Could you check a few things on this drawing? It's one solid part, dimensions in mm from its lowest x, y, z. A direction names the side the tool comes from. Round coordinates to 2 decimals unless told otherwise and drop trailing zeros. Order: outer loops, then holes, each group sorted by start corner. A loop starts at its lowest first (then second) coordinate and runs counter-clockwise, first axis right, second up. Notation, with made-up numbers: (64, 31.25) -> (79, 31.25) arc R30 cw to (79, 67.25) -> close; hole circle Ø6 at (35, 22). An arc over 180 degrees is marked (long way). Use a Markdown table: item, result. Add a question column.
(1) If I drill on probe 1 along X at (y, z) = (5.75, 6.5); probe 2 along X at (y, z) = (0.8, 5) (1 decimal); probe 3 along X at (y, z) = (0.55, 30) (1 decimal), over which ranges is the centre line in solid material (lowest first)?
(2) I want a section at B-B, the plane y = 8.25. Please give me the cut outline in (x, z).
(3) Thinking about a two-plate mould opening in X: for the marked faces 5, 6, 7 and 8, which applies, pulls with the +X half, pulls with the -X half, needs draft (parallel to the pull), parting line crosses it, or undercut?
(4) On a 3-axis mill with a long thin cutter (end or side, diameter ignored), from which of +Z, -Z, +X, -X, +Y, -Y can I reach the whole of each face in a straight line? I mean the marked faces 1, 2, 3 and 4. Say none if no direction works.
(5) I want a section at D-D, the plane z = 5. Please give me the cut outline in (x, y) (1 decimal).
(6) I want a section at C-C, the plane z = 30. Please give me the cut outline in (x, y) (1 decimal).
(7) I want a section at A-A, the plane z = 26. Please give me the cut outline in (x, y), then the cut area to 3 significant figures.
(8) I'm going to push flat-ended pins straight in: P1, Ø4.5, axis at x = 4.73, z = 5, coming from the +Y side; P2, Ø9.5, axis at y = 12, z = 17, coming from the +X side; P3, Ø14.5, axis at x = 27, z = 7.5, coming from the -Y side. Where does each tip first touch, or does it pass through?
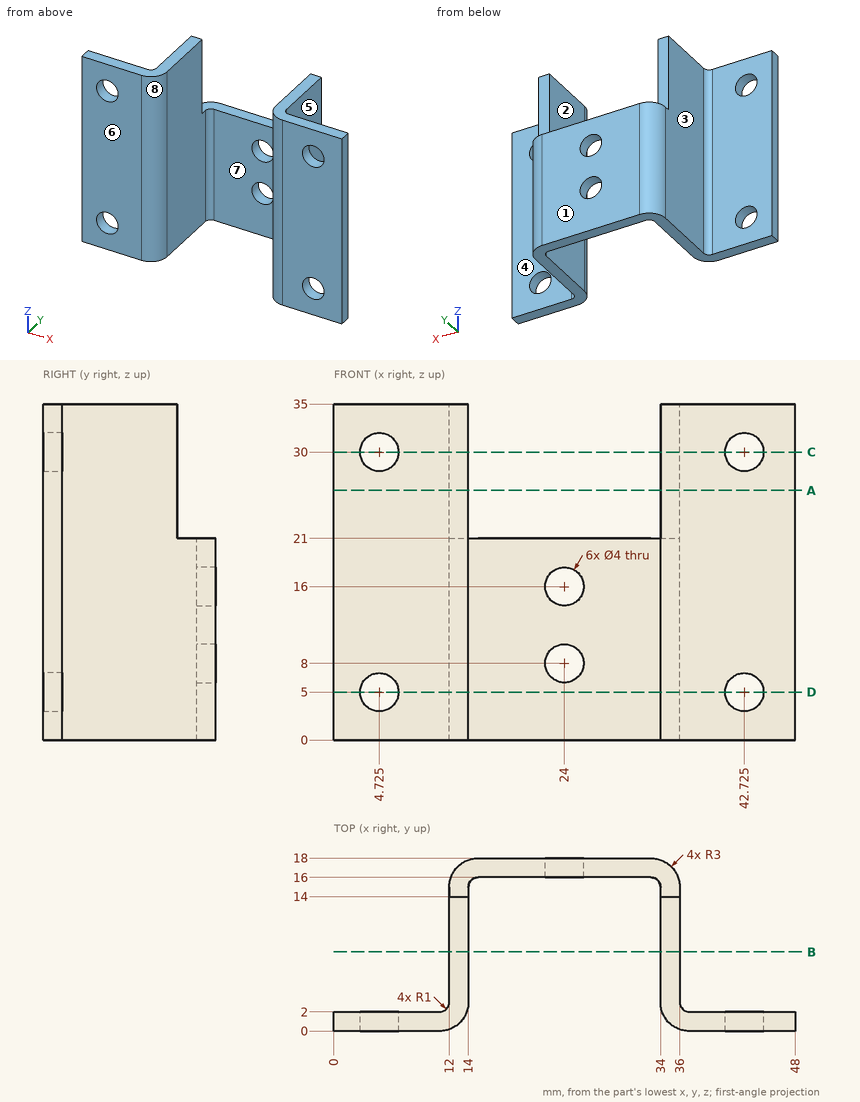
Taken from the geometry:
| question | item | result |
|---|---|---|
| 1 | probe 1 | x = 12 to 14, 34 to 36 |
| 1 | probe 2 | x = 0 to 2.7, 6.7 to 13, 35 to 40.7, 44.7 to 48 |
| 1 | probe 3 | x = 0 to 2.7, 6.7 to 12.7, 35.3 to 40.7, 44.7 to 48 |
| 2 | outline | (12, 0) -> (14, 0) -> (14, 35) -> (12, 35) -> close; (34, 0) -> (36, 0) -> (36, 35) -> (34, 35) -> close |
| 3 | face 5 | pulls with the +X half |
| 3 | face 6 | needs draft |
| 3 | face 7 | undercut |
| 3 | face 8 | undercut |
| 4 | face 1 | +Z, -Z, +X, -X, +Y |
| 4 | face 2 | +Z, -Z, -Y |
| 4 | face 3 | +Z, -Z, -X, +Y |
| 4 | face 4 | +Z, -Z, +X, +Y |
| 5 | outline | (0, 0) -> (2.7, 0) -> (2.7, 2) -> (0, 2) -> close; (6.7, 0) -> (11, 0) arc R3 ccw to (14, 3) -> (14, 15) arc R1 cw to (15, 16) -> (33, 16) arc R1 cw to (34, 15) -> (34, 3) arc R3 ccw to (37, 0) -> (40.7, 0) -> (40.7, 2) -> (37, 2) arc R1 cw to (36, 3) -> (36, 15) arc R3 ccw to (33, 18) -> (15, 18) arc R3 ccw to (12, 15) -> (12, 3) arc R1 cw to (11, 2) -> (6.7, 2) -> close; (44.7, 0) -> (48, 0) -> (48, 2) -> (44.7, 2) -> close |
| 6 | outline | (0, 0) -> (2.7, 0) -> (2.7, 2) -> (0, 2) -> close; (6.7, 0) -> (11, 0) arc R3 ccw to (14, 3) -> (14, 14) -> (12, 14) -> (12, 3) arc R1 cw to (11, 2) -> (6.7, 2) -> close; (34, 3) arc R3 ccw to (37, 0) -> (40.7, 0) -> (40.7, 2) -> (37, 2) arc R1 cw to (36, 3) -> (36, 14) -> (34, 14) -> close; (44.7, 0) -> (48, 0) -> (48, 2) -> (44.7, 2) -> close |
| 7 | outline | (0, 0) -> (11, 0) arc R3 ccw to (14, 3) -> (14, 14) -> (12, 14) -> (12, 3) arc R1 cw to (11, 2) -> (0, 2) -> close; (34, 3) arc R3 ccw to (37, 0) -> (48, 0) -> (48, 2) -> (37, 2) arc R1 cw to (36, 3) -> (36, 14) -> (34, 14) -> close |
| 7 | area | 101 mm2 |
| 8 | P1 | stops at y = 2 |
| 8 | P2 | stops at x = 36 |
| 8 | P3 | stops at y = 1.8 |
